Read the model definition and answer for the solid it produces. Units are mm, in the model's axes. Face numbers are marked on the shaded views. Give positions to 0.01 mm unless a question says otherwise; leave off trailing zeros. Loops run counter-clockwise (first coordinate to the right, second up) from the corner with the lowest first, then second, coordinate; pieces in that order, holes last. Notation, with made-up numbers: (19.25, 14.25) - (76.25, 14.25) arc R13 ccw to (76.25, 39.25) - close; hole circle Ø1 at (82, -15). An arc over 180 degrees is marked (long way). Put each result on its own line as item: value. Start each with the question number.
1. A cutting plane is placed at A-A, the plane y = 0. Determine the outline of the cut face in (x, z).
2. Given pin 1 Ø2 at (y, z) = (28.5, 2) entering from +X; pin 2 Ø1.5 at (y, z) = (16.5, 5.5) entering from +X; pin 3 Ø1 at (x, z) = (-28.5, 2) entering from +Y, each flat-ended and moving along its own axis, determine where each tip first touches the part or whether it passes through.
3. Consider L1, parallel to Y at x = 0, z = 6.75; L2, parallel to X at y = 9, z = 4; L3, parallel to Y at x = -28, z = 8.5. Determine where each line is inside the solid, lowest interval first. Write a range as from..to.
4. A cutting plane is placed at C-C, the plane z = 7.25. Determine the outline of the cut face in (x, y), plus the area to 3 significant figures.
5. For a pull along X with two mould halves and no side action, classify the marked faces 1, 2 and 3 as released by +X, released by -X, zero draft, split by the parting line, or undercut.
```python
from build123d import *

# Parameters (mm, degrees)
ESQUISSE1_R             = 37
ESQUISSE1_R_2           = 35
BOSS_EXTRU_1_DEPTH      = 10
ESQUISSE3_R             = 40
BOSS_EXTRU_2_DEPTH      = 2
ENL_V_START             = -2
ESQUISSE4_R             = 35
ENL_V_MAT_EXTRU_1_DEPTH = 2


with BuildPart() as part:
    # Esquisse1 → Boss.-Extru.1 (new body)
    with BuildSketch(Plane.XY):
        Circle(ESQUISSE1_R)
        Circle(ESQUISSE1_R_2, mode=Mode.SUBTRACT)
    extrude(amount=BOSS_EXTRU_1_DEPTH)

    # Esquisse3 → Boss.-Extru.2 (add)
    with BuildSketch(Plane.XY):
        Circle(ESQUISSE3_R)
    extrude(amount=BOSS_EXTRU_2_DEPTH)

    # Esquisse4 → Enlèv. mat.-Extru.1 (cut)
    with BuildSketch(Plane.XY.offset(2).offset(ENL_V_START)):
        Circle(ESQUISSE4_R)
    extrude(amount=ENL_V_MAT_EXTRU_1_DEPTH, mode=Mode.SUBTRACT)


solid = part.part
```
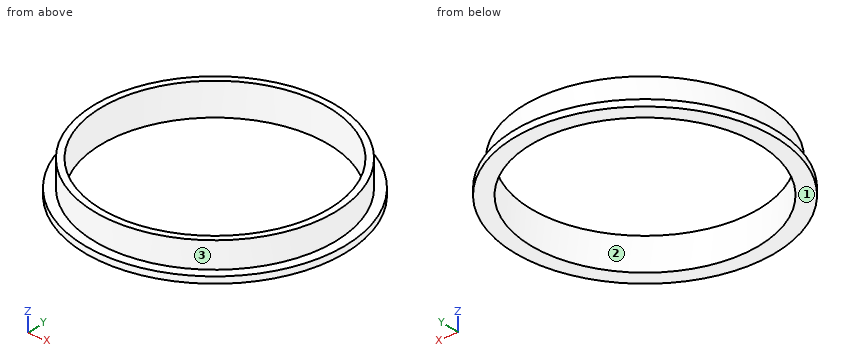
Return value:
1. outline: (-40, 0) - (-35, 0) - (-35, 10) - (-37, 10) - (-37, 2) - (-40, 2) - close; (35, 0) - (40, 0) - (40, 2) - (37, 2) - (37, 10) - (35, 10) - close
2. pin 1: stops at x = 29.05
2. pin 2: stops at x = 33.48
2. pin 3: stops at y = 28.57
3. L1: y = -37..-35, 35..37
3. L2: x = -35.89..-33.82, 33.82..35.89
3. L3: y = -24.19..-21, 21..24.19
4. outline: circle Ø74 at (0, 0); hole circle Ø70 at (0, 0)
4. area: 452 mm2
5. face 1: zero draft
5. face 2: undercut
5. face 3: split by the parting line
